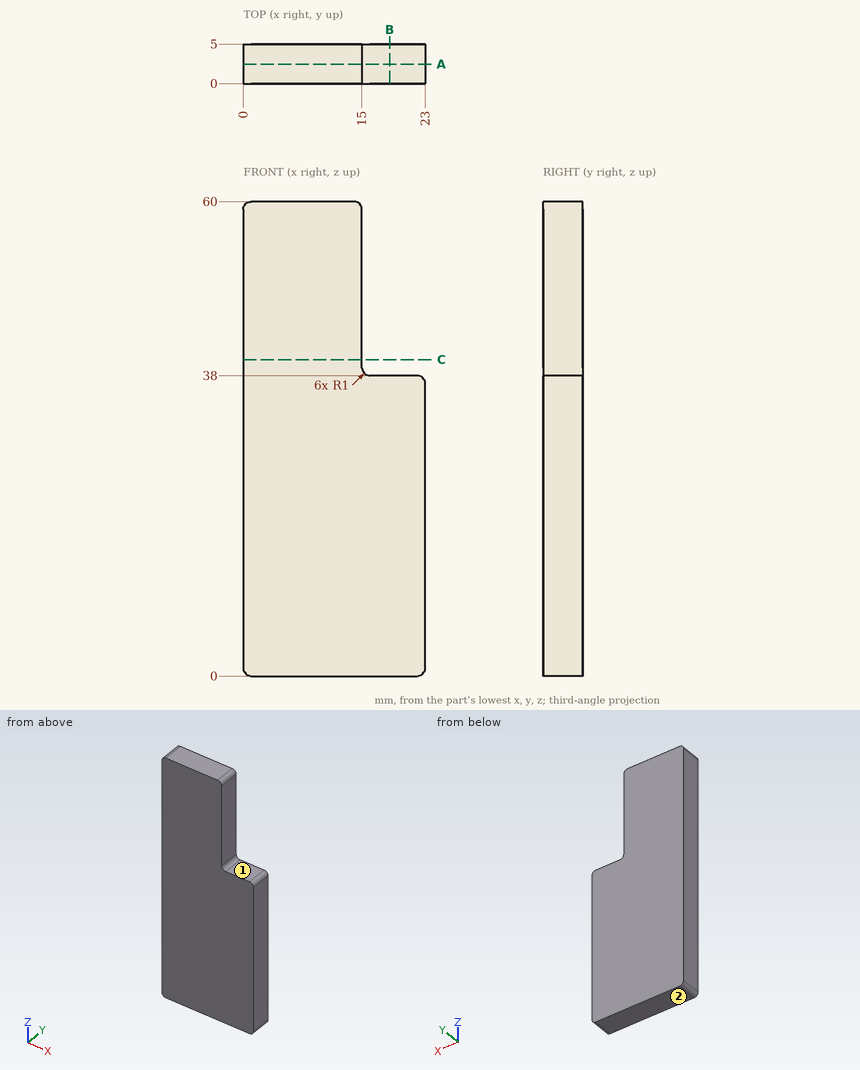
Design review of the part shown in the three views and the two pictorial views. Dimensions are in mm from the part's minimum x, y and z. A direction names the side the tool comes from. Round coordinates to 2 decimals unless told otherwise and drop trailing zeros. Loops run counter-clockwise (first coordinate to the right, second up) from the corner with the lowest first, then second, coordinate; pieces in that order, holes last. Notation, with made-up numbers: (52.25, 24.25) -> (102.25, 24.25) arc R22 cw to (102.25, 36.25) -> close; hole circle Ø6 at (19.25, 88.5). An arc over 180 degrees is marked (long way). Return JSON: item names as keys, results as strings.
(1) Add section C-C on z = 40. Write out the cut boundary in (x, y), plus the area to 3 significant figures.
Solved:
{"outline": "(0, 0) -> (15, 0) -> (15, 5) -> (0, 5) -> close", "area": "75.0 mm2"}
(2) For the marked faces 1 and 2, list the 3-axis set-ups (+Z, -Z, +X, -X, +Y, -Y) from which the entire face can be reached by the end or side of a thin tool; tool diameter is ignored.
Solved:
{"face 1": "+Z, +X, +Y, -Y", "face 2": "-Z, +X, -X, +Y, -Y"}
(3) For line 1 (Z direction, x = 17, y = 2.5); line 2 (X direction, y = 1.65, z = 55), list the stretches that pass through material, from the lowest coordinate up.
Solved:
{"line 1": "0 to 38", "line 2": "0 to 15"}
(4) Add section B-B on x = 18.5. Write out the cut boundary in (y, z), plus the area to 3 significant figures.
Solved:
{"outline": "(0, 0) -> (5, 0) -> (5, 38) -> (0, 38) -> close", "area": "190 mm2"}
(5) Add section A-A on y = 2.45. Write out the cut boundary in (x, z).
Solved:
{"outline": "(0, 1) arc R1 ccw to (1, 0) -> (22, 0) arc R1 ccw to (23, 1) -> (23, 37) arc R1 ccw to (22, 38) -> (16, 38) arc R1 cw to (15, 39) -> (15, 59) arc R1 ccw to (14, 60) -> (1, 60) arc R1 ccw to (0, 59) -> close"}
(6) For pin 1 (1.5 mm diameter, centred on x = 19.5, y = 2.5, fed in from +Z), flat-tipped, find the tip position at first contact; note if it passes through.
Solved:
{"pin 1": "z = 38"}
